```python
from build123d import *

# Parameters (mm, degrees)
F0_R      = 21.5
F1_DEPTH  = 40
F2_R      = 5
F3_R      = 21.5
F4_DEPTH  = 40
F5_SIZE2  = 7.5
F5_SIZE   = 40
F6_DEPTH  = 10
F7_R      = 10
F10_R     = 4.9
F11_DEPTH = 75
F12_R     = 16.5
F13_DEPTH = 5
F14_R     = 3.1
F15_DEPTH = 85.001


with BuildPart() as f1:
    # F0 (on Top) → F1 (new body)
    with BuildSketch(Plane.XY):
        Circle(F0_R)
    extrude(amount=F1_DEPTH)

    # F2
    f2_edges = [f1.edges().sort_by_distance(p)[0] for p in [
        (-21.5, 0, 40),
    ]]
    fillet(f2_edges, radius=F2_R)

    # F3 (on face) → F4 (join)
    with BuildSketch(Plane(origin=(0, 0, 0), x_dir=(1, 0, 0), z_dir=(0, 0, -1))):
        Circle(F3_R)
    extrude(amount=F4_DEPTH)

    # F5
    f5_edges = [f1.edges().sort_by_distance(p)[0] for p in [
        (-21.5, 0, -40),
    ]]
    chamfer(f5_edges, length=F5_SIZE, length2=F5_SIZE2)

    # F6 (add): a face of the model
    f6_faces = [f1.faces().sort_by_distance(p)[0] for p in [
        (0, 0, -40),
    ]]
    extrude(f6_faces, amount=F6_DEPTH)

    # F7
    f7_edges = [f1.edges().sort_by_distance(p)[0] for p in [
        (-21.5, 0, 0),
    ]]
    fillet(f7_edges, radius=F7_R)

    # F8 (on Right) → F9 (revolve, cut)
    with BuildSketch(Plane.YZ):
        Polygon((-7.5, -40.5), (-17.4298945979, -40.5), (-17.4298945979, -47.5), (-17.4298945979, -53.659953177), (-10, -53.659953177), (-10, -47.5), (-7.5, -47.5), align=None)
    revolve(axis=Axis((0, 0, -53.4000843763), (0, 0, -1)), mode=Mode.SUBTRACT)

    # F10 (on face) → F11 (cut)
    with BuildSketch(Plane(origin=(0, 0, -50), x_dir=(1, 0, 0), z_dir=(0, 0, -1))):
        Circle(F10_R)
    extrude(amount=-F11_DEPTH, mode=Mode.SUBTRACT)

    # F12 (on face) → F13 (cut)
    with BuildSketch(Plane.XY.offset(40)):
        Circle(F12_R)
    extrude(amount=-F13_DEPTH, mode=Mode.SUBTRACT)

    # F14 (on face) → F15 (cut, through all)
    with BuildSketch(Plane.XY.offset(35)):
        Circle(F14_R)
    extrude(amount=-F15_DEPTH, mode=Mode.SUBTRACT)


solid = f1.part
```
Design review of the part built by this model. Coordinates are the model's own, in mm. A direction names the side the tool comes from. Give positions to 0.01 mm unless a question says otherwise; leave off trailing zeros. Loops run counter-clockwise (first coordinate to the right, second up) from the corner with the lowest first, then second, coordinate; pieces in that order, holes last. Notation, with made-up numbers: (34.25, 65.25) -> (45.25, 65.25) arc R21 ccw to (45.25, 87.25) -> close; hole circle Ø7 at (31.5, -12). An arc over 180 degrees is marked (long way). One line per item, written item: value.
Q1. For L1, parallel to Y at x = 0, z = 3.5; L2, parallel to Y at x = 0, z = 36.3, list the stretches that pass through material, from the lowest coordinate up.
Numbers:
L1: y = -21.5 to -4.9, 4.9 to 21.5
L2: y = -21.33 to -16.5, 16.5 to 21.33
Q2. For pin 1 Ø3 at (x, y) = (1.5, 1.5) entering from -Z; pin 2 Ø1.5 at (x, y) = (8, 12.5) entering from +Z; pin 3 Ø12.5 at (x, y) = (0, 0) entering from -Z; pin 4 Ø2 at (y, z) = (-3, 10) entering from -X, all flat-tipped, find the tip position at first contact; note any pin that passes through.
Numbers:
pin 1: stops at z = 25
pin 2: stops at z = 35
pin 3: stops at z = -50
pin 4: stops at x = -21.41
Q3. Machinability: for faces 1 (the flat face through (6, 6, -40.5)), 2 (the cylindrical face through (-1.062, 4.783, -13.025)), 3 (the cylindrical face through (-2.799, -21.317, 18.203)), 4 (the cylindrical face through (15.24, -6.32, 37.53)), which of the approach directions +Z, -Z, +X, -X, +Y, -Y give a long, thin tool a straight path to every point of the face, cutting with its end or side? Answer none if there is none.
Numbers:
face 1: none
face 2: -Z
face 3: +Z, -Z
face 4: +Z
Q4. Draft analysis for pull direction Y (two halves, no side actions). For faces 5 (the cylindrical face through (12.932, 5.362, -40.246)), 6 (the flat face through (-0.2, -3.4, 35)), 7 (the flat face through (2, -5, -50)), state which applies: pulls with the +Y half, pulls with the -Y half, needs draft (parallel to the pull), parting line crosses it, or undercut.
Numbers:
face 5: parting line crosses it
face 6: undercut
face 7: needs draft
Q5. We need section B-B on z = 20. Give the boundary of the cut face in (x, y).
Numbers:
outline: circle Ø43 at (0, 0); hole circle Ø9.8 at (0, 0)
Q6. We need section A-A on z = -43.5. Give the boundary of the cut face in (x, y), and give its area (3 significant figures).
Numbers:
outline: circle Ø15 at (0, 0); hole circle Ø9.8 at (0, 0)
area: 101 mm^2
